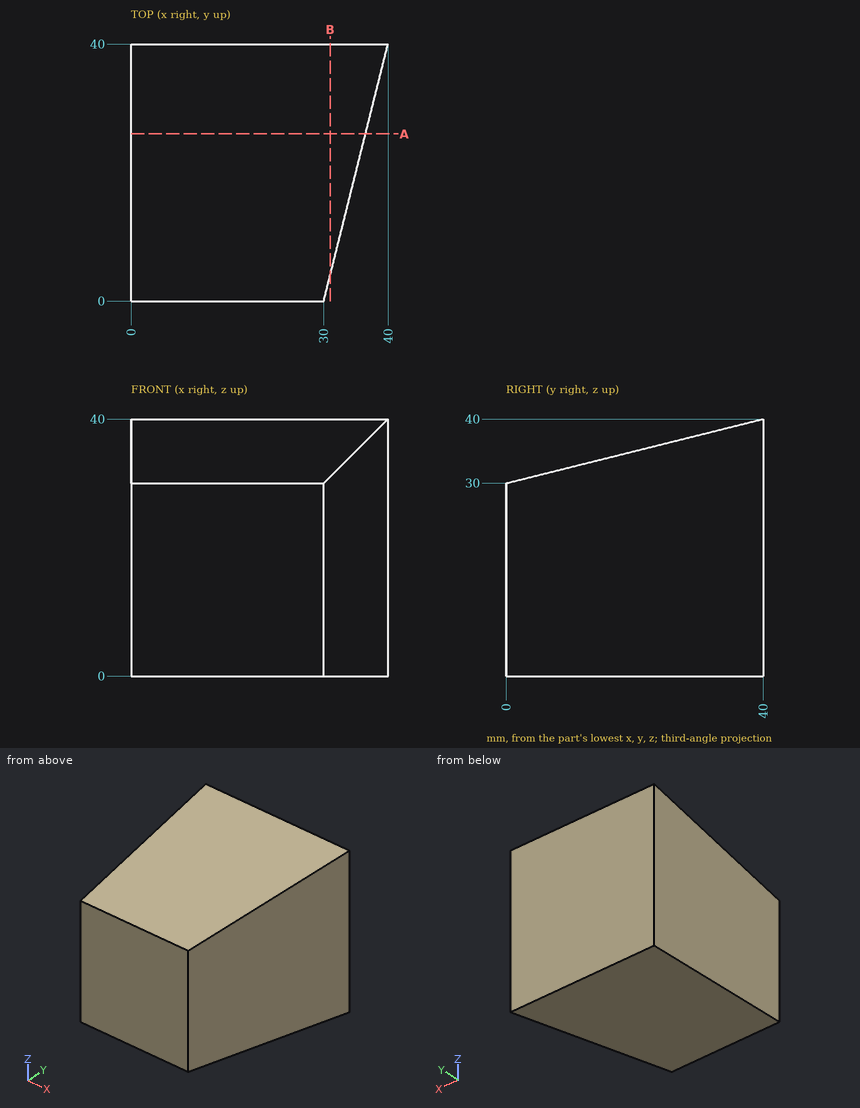
Drawing for the job (mm, zero at the part's lowest x, y, z). Round coordinates to 2 decimals unless told otherwise and drop trailing zeros. Write each loop counter-clockwise with the first axis right and the second up, starting at its lowest first coordinate (ties: lowest second). Pieces come first, ordered by that corner, then holes. Notation, with made-up numbers: M 1.5,7.25 L 25.5,7.25 A14 ccw 25.5,26.25 Z; hole C 85,70.5 d1. An arc over 180 degrees is marked long. Answer as a JSON object with one key per item and string values. Group by question number.
(1) Flat gauge pins, fed straight in: pin 1 (6 mm diameter, centred on y = 5, z = 31, fed in from +X); pin 2 (4 mm diameter, centred on x = 33.5, y = 13.5, fed in from -Z); pin 3 (2 mm diameter, centred on y = 11.5, z = 4.5, fed in from +X) (3 decimals); pin 4 (1 mm diameter, centred on y = 32, z = 8, fed in from +X) (3 decimals). Where does each tip first touch, or does it go through?
(2) Cut at A-A (y = 26). Give the cut face in (x, z), and give its area (3 significant figures).
(3) Cut at B-B (x = 31). Give the cut face in (y, z).
(4) Drill centre lines: L1, parallel to Z at x = 30.5, y = 22.5 (3 decimals); L2, parallel to X at y = 18.5, z = 12 (3 decimals); L3, parallel to X at y = 17, z = 12. Where is each one in solid material? Low to high.
Responses:
{
 "1": {"pin 1": "stops at x = 32", "pin 2": "stops at z = 0", "pin 3": "stops at x = 33.125", "pin 4": "stops at x = 38.125"},
 "2": {"outline": "M 0,0 L 36.5,0 L 36.5,36.5 L 0,36.5 Z", "area": "1,330 mm2"},
 "3": {"outline": "M 4,0 L 40,0 L 40,40 L 4,31 Z"},
 "4": {"L1": "z = 0 to 35.625", "L2": "x = 0 to 34.625", "L3": "x = 0 to 34.25"}
}
